Read the model definition and answer for the solid it produces. Units are mm, in the model's axes. Round coordinates to 2 decimals unless told otherwise and drop trailing zeros. Loops run counter-clockwise (first coordinate to the right, second up) from the corner with the lowest first, then second, coordinate; pieces in that order, holes last. Notation, with made-up numbers: M 20,19 L 77,19 A13 ccw 77,41 Z; hole C 84,-30 d5. An arc over 180 degrees is marked long. Write each question's results on one line, items separated by ' | '.
from build123d import *

# Parameters (mm, degrees)
SKETCH_1_R      = 28
SKETCH_1_R_2    = 6
EXTRUDE_1_DEPTH = 3


with BuildPart() as part:
    # 草图1 → 凸台-拉伸1 (new body)
    with BuildSketch(Plane.XY):
        Circle(SKETCH_1_R)
        Circle(SKETCH_1_R_2, mode=Mode.SUBTRACT)
        with BuildLine():
            Line((-13, 22.516660498), (-4, 6.92820323))
            ThreePointArc((-4, 6.92820323), (0, 8), (4, 6.92820323))
            Line((4, 6.92820323), (13, 22.516660498))
            ThreePointArc((13, 22.516660498), (0, 26), (-13, 22.516660498))
        make_face(mode=Mode.SUBTRACT)
        with BuildLine():
            Line((-13, -22.516660498), (-4, -6.92820323))
            ThreePointArc((-4, -6.92820323), (-6.92820323, -4), (-8, 0))
            Line((-8, 0), (-26, 0))
            ThreePointArc((-26, 0), (-22.516660498, -13), (-13, -22.516660498))
        make_face(mode=Mode.SUBTRACT)
        with BuildLine():
            Line((13, -22.516660498), (4, -6.92820323))
            ThreePointArc((4, -6.92820323), (6.92820323, -4), (8, 0))
            Line((8, 0), (26, 0))
            ThreePointArc((26, 0), (22.516660498, -13), (13, -22.516660498))
        make_face(mode=Mode.SUBTRACT)
    extrude(amount=EXTRUDE_1_DEPTH)


solid = part.part
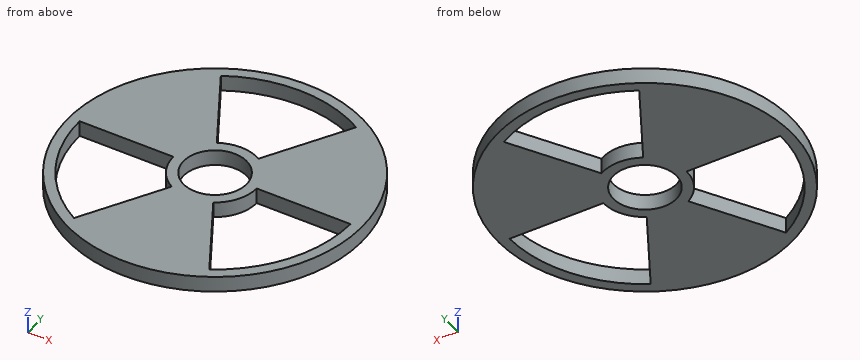
Item 1: The part is cut by section D-D (x = 24). Determine the outline of the cut face in (y, z), plus the area to 3 significant figures.
Outcome:
outline: M -14.42,0 L -10,0 L -10,3 L -14.42,3 Z; M 0,0 L 14.42,0 L 14.42,3 L 0,3 Z | area: 56.5 mm2
Item 2: The part is cut by section B-B (x = 0). Determine the outline of the cut face in (y, z).
Outcome:
outline: M -28,0 L -6,0 L -6,3 L -28,3 Z; M 6,0 L 8,0 L 8,3 L 6,3 Z; M 26,0 L 28,0 L 28,3 L 26,3 Z
Item 3: The part is cut by section C-C (y = 19.5). Determine the outline of the cut face in (x, z), plus the area to 3 significant figures.
Outcome:
outline: M -20.09,0 L -11.26,0 L -11.26,3 L -20.09,3 Z; M 11.26,0 L 20.09,0 L 20.09,3 L 11.26,3 Z | area: 53.0 mm2
Item 4: Flat-ended cylindrical pins translate along their axes: pin 1 (10 mm diameter, centred on x = -17.5, y = -10, fed in from -Z); pin 2 (1 mm diameter, centred on y = 3.5, z = 2.5, fed in from +X); pin 3 (1 mm diameter, centred on x = -14.5, z = 1.5, fed in from +Y); pin 4 (0.9 mm diameter, centred on x = 15, z = 1, fed in from -Y). Find the tip coordinate at first contact, or state that the pin passes through.
Outcome:
pin 1: passes through | pin 2: stops at x = 27.84 | pin 3: stops at y = 24.25 | pin 4: stops at y = -23.92
Item 5: Straight lines are drawn through the part: line 1 (Y direction, x = 0, z = 1.4); line 2 (Y direction, x = 8.5, z = 1.3); line 3 (X direction, y = -22, z = 2.7). For each, find the intervals that lie inside material, in ascending order.
Outcome:
line 1: y = -28 to -6, 6 to 8, 26 to 28 | line 2: y = -26.68 to -14.72, 0 to 14.72, 24.57 to 26.68 | line 3: x = -17.32 to -13.86, -12.7 to 12.7, 13.86 to 17.32
Item 6: The part is cut by section A-A (z = 0.8). Determine the outline of the cut face in (x, y).
Outcome:
outline: C 0,0 d56; hole M -26,0 A26 ccw -13,-22.52 L -4,-6.93 A8 cw -8,0 Z; hole M -13,22.52 L -4,6.93 A8 cw 4,6.93 L 13,22.52 A26 ccw Z; hole C 0,0 d12; hole M 4,-6.93 L 13,-22.52 A26 ccw 26,0 L 8,0 A8 cw Z
